CAD build for the part. Positions are in the model's coordinates, mm. A direction names the side the tool comes from. Give positions to 0.01 mm unless a question says otherwise; leave off trailing zeros. Order: outer loops, then holes, each group sorted by start corner. A loop starts at its lowest first (then second) coordinate and runs counter-clockwise, first axis right, second up. Notation, with made-up numbers: (16, 0) -> (73, 0) arc R16 cw to (73, 19) -> close; hole circle Ø4 at (45, 81). An arc over 180 degrees is marked (long way). Answer as CSV lines item,"result".
Autodesk Inventor part; units mm, degrees
ref_plane "YZ Plane" through (0, 0, 0) normal (1, 0, 0) x (0, 1, 0)
ref_plane "XZ Plane" through (0, 0, 0) normal (0, 1, 0) x (-1, 0, 0)
ref_plane "XY Plane" through (0, 0, 0) normal (0, 0, 1) x (1, 0, 0)
sketch "スケッチ1" plane through (0, 0, 0) normal (0, 0, 1) x (1, 0, 0)
  line L0 (0, 0) -> (3, 0)
  line L1 (3, 0) -> (3, -15)
  line L2 (3, -15) -> (0, -15)
  line L3 (0, -15) -> (0, 0)
  line L4 (-15, 0) -> (-12, 0)
  line L5 (-12, 0) -> (-12, -15)
  line L6 (-12, -15) -> (-15, -15)
  line L7 (-15, -15) -> (-15, 0)
  line L8 (-26.0926, 3) -> (-139.0635, -55.2952)
  line L9 (7, 3) -> (7, -18)
  line L10 (-7.8217, -18) -> (-133.786, -83)
  circle A0 centre (-135, -78) radius 2
  circle A1 centre (-150, -78) radius 2
  line L11 (-150, -78) -> (-135, -78) construction
  arc A2 (-154.0422, -75.0571) -> (-150, -83) centre (-150, -78) ccw
  line L12 (-140.638, -56.6456) -> (-154.0422, -75.0571)
  circle A3 centre (-15, -1.05) radius 1.05
  circle A4 centre (-15, -13.95) radius 1.05
  circle A5 centre (-12, -13.95) radius 1.05
  circle A6 centre (-12, -1.05) radius 1.05
  circle A7 centre (0, -1.05) radius 1.05
  circle A8 centre (3, -1.05) radius 1.05
  circle A9 centre (0, -13.95) radius 1.05
  circle A10 centre (3, -13.95) radius 1.05
  arc A11 (-139.0635, -55.2952) -> (-140.638, -56.6456) centre (-137, -59.2941) ccw
  circle A12 centre (-100.7273, -60.8773) radius 4.5 construction
  circle A13 centre (-81, -30.3971) radius 4.5 construction
  circle A14 centre (-44.7273, -31.9802) radius 4.5 construction
  circle A15 centre (-25, -1.5) radius 4.5 construction
  circle A16 centre (-137, -59.2941) radius 1.5
  circle A17 centre (-100.7273, -60.8773) radius 1.5
  circle A18 centre (-81, -30.3971) radius 1.5
  circle A19 centre (-44.7273, -31.9802) radius 1.5
  circle A20 centre (-25, -1.5) radius 1.5
  circle A21 centre (-4.5, -7.5) radius 1.5
  circle A22 centre (-19.5, -7.5) radius 1.5
  line L13 (-26.0926, 3) -> (7, 3)
  line L14 (-7.8217, -18) -> (7, -18)
  line L15 (-150, -83) -> (-133.786, -83)
  circle A23 centre (-135, -78) radius 5
  line L16 (-25, -1.5) -> (-44.7273, -31.9802) construction
  line L17 (-44.7273, -31.9802) -> (-81, -30.3971) construction
  line L18 (-81, -30.3971) -> (-100.7273, -60.8773) construction
  line L19 (-100.7273, -60.8773) -> (-137, -59.2941) construction
  point P0 (0, -12.9)
  point P1 (0, -2.1)
  point P2 (3, -2.1)
  point P3 (3, -12.9)
  point P4 (-12, -2.1)
  point P5 (-12, -12.9)
  point P6 (-15, -12.9)
  point P7 (-15, -2.1)
  dimension "d0" = 3
  dimension "d1" = 15
  dimension "d2" = 3
  dimension "d3" = 15
  dimension "d4" = 12
  dimension "d5" = 4
  dimension "d6" = 4
  dimension "d7" = 15
  dimension "d8" = 4
  dimension "d12" = 3
  dimension "d13" = 2.1
  dimension "d14" = 2.1
  dimension "d15" = 2.1
  dimension "d16" = 2.1
  dimension "d17" = 2.1
  dimension "d18" = 2.1
  dimension "d19" = 2.1
  dimension "d20" = 2.1
  dimension "d23" = 9
  dimension "d24" = 9
  dimension "d25" = 9
  dimension "d26" = 9
  dimension "d27" = 9
  dimension "d28" = 3
  dimension "d29" = 3
  dimension "d30" = 3
  dimension "d31" = 3
  dimension "d32" = 3
  dimension "d33" = 10
  dimension "d34" = 3
  dimension "d35" = 3
  dimension "d36" = 4.5
  dimension "d37" = 4.5
  dimension "d38" = 7.5
  dimension "d39" = 7.5
  dimension "d60" = 120
  dimension "d61" = 3
  dimension "d62" = 3
  dimension "d63" = 3
  dimension "d64" = 60
extrude "押し出し1" add sketch "スケッチ1" along normal blind 3
sketch "スケッチ3" plane through (0, 0, 3) normal (0, 0, 1) x (1, 0, 0)
  line L0 (-150, -83) -> (-133.786, -83)
  line L1 (-133.786, -83) -> (-7.8217, -18)
  line L2 (-7.8217, -18) -> (7, -18)
  line L3 (7, -18) -> (7, 3)
  line L4 (7, 3) -> (-26.0926, 3)
  line L5 (-26.0926, 3) -> (-139.0635, -55.2952)
  arc A0 (-139.0635, -55.2952) -> (-140.638, -56.6456) centre (-137, -59.2941) ccw
  line L6 (-140.638, -56.6456) -> (-154.0422, -75.0571)
  arc A1 (-154.0422, -75.0571) -> (-150, -83) centre (-150, -78) ccw
  circle A2 centre (-19.5, -7.5) radius 1.5
  circle A3 centre (-25, -1.5) radius 1.5
  circle A4 centre (-44.7273, -31.9802) radius 1.5
  circle A5 centre (-81, -30.3971) radius 1.5
  circle A6 centre (-100.7273, -60.8773) radius 1.5
  circle A7 centre (-137, -59.2941) radius 1.5
  arc A8 (3, -2.1) -> (3, 0) centre (3, -1.05) ccw
  line L7 (3, -2.1) -> (3, -12.9)
  arc A9 (3, -15) -> (3, -12.9) centre (3, -13.95) ccw
  line L8 (3, -15) -> (0, -15)
  arc A10 (0, -12.9) -> (0, -15) centre (0, -13.95) ccw
  line L9 (0, -12.9) -> (0, -2.1)
  arc A11 (0, 0) -> (0, -2.1) centre (0, -1.05) ccw
  line L10 (0, 0) -> (3, 0)
  circle A12 centre (-135, -78) radius 2
  line L11 (-12, -2.1) -> (-12, -12.9)
  arc A13 (-12, -15) -> (-12, -12.9) centre (-12, -13.95) ccw
  line L12 (-12, -15) -> (-15, -15)
  arc A14 (-15, -12.9) -> (-15, -15) centre (-15, -13.95) ccw
  line L13 (-15, -12.9) -> (-15, -2.1)
  arc A15 (-15, 0) -> (-15, -2.1) centre (-15, -1.05) ccw
  line L14 (-15, 0) -> (-12, 0)
  arc A16 (-12, -2.1) -> (-12, 0) centre (-12, -1.05) ccw
  circle A17 centre (-4.5, -7.5) radius 1.5
  circle A18 centre (-150, -78) radius 2
  line L15 (-137.6878, -57.9612) -> (-25.3642, 0)
  line L16 (-25.3642, 0) -> (4, 0)
  line L17 (4, 0) -> (4, -15)
  line L18 (4, -15) -> (-8.5501, -15)
  line L19 (-8.5501, -15) -> (-134.5144, -80)
  line L20 (-134.5144, -80) -> (-150, -80)
  arc A19 (-151.6169, -76.8229) -> (-150, -80) centre (-150, -78) ccw
  line L21 (-151.6169, -76.8229) -> (-138.2127, -58.4113)
  arc A20 (-137.6878, -57.9612) -> (-138.2127, -58.4113) centre (-137, -59.2941) ccw
  circle A21 centre (-81, -30.3971) radius 4.5
  circle A22 centre (-100.7273, -60.8773) radius 4.5
  circle A23 centre (-137, -59.2941) radius 4.5
  circle A24 centre (-44.7273, -31.9802) radius 4.5
  circle A25 centre (-19.5, -7.5) radius 4.5
  line L22 (-9, -11.2292) -> (-9, -3.7708)
  arc A26 (-9, -3.7708) -> (-12, 3) centre (-12, -1.05) ccw
  line L23 (-12, 3) -> (-15, 3)
  arc A27 (-15, 3) -> (-18, -3.7708) centre (-15, -1.05) ccw
  line L24 (-18, -3.7708) -> (-18, -11.2292)
  arc A28 (-18, -11.2292) -> (-15, -18) centre (-15, -13.95) ccw
  line L25 (-15, -18) -> (-12, -18)
  arc A29 (-12, -18) -> (-9, -11.2292) centre (-12, -13.95) ccw
  circle A30 centre (-25, -1.5) radius 4.5
  line L26 (-3, -3.7708) -> (-3, -11.2292)
  arc A31 (-3, -11.2292) -> (0, -18) centre (0, -13.95) ccw
  line L27 (0, -18) -> (3, -18)
  arc A32 (3, -18) -> (6, -11.2292) centre (3, -13.95) ccw
  line L28 (6, -11.2292) -> (6, -3.7708)
  arc A33 (6, -3.7708) -> (3, 3) centre (3, -1.05) ccw
  line L29 (3, 3) -> (0, 3)
  arc A34 (0, 3) -> (-3, -3.7708) centre (0, -1.05) ccw
  circle A35 centre (-4.5, -7.5) radius 4.6
  circle A36 centre (-135, -78) radius 5
  circle A37 centre (-150, -78) radius 5
  line L30 (-135, -73) -> (-150, -73)
  circle A38 centre (-137, -59.2941) radius 1.5
  line L31 (-137, -59.2941) -> (-100.7273, -60.8773) construction
  line L32 (-137.0654, -60.7927) -> (-100.7927, -62.3759)
  line L33 (-100.6619, -59.3787) -> (-136.9346, -57.7956)
  arc A39 (-136.9346, -57.7956) -> (-137.0654, -60.7927) centre (-137, -59.2941) ccw
  arc A40 (-100.7927, -62.3759) -> (-100.6619, -59.3787) centre (-100.7273, -60.8773) ccw
  line L34 (-81, -30.3971) -> (-100.7273, -60.8773) construction
  line L35 (-82.2593, -29.5821) -> (-101.9866, -60.0623)
  line L36 (-99.4681, -61.6923) -> (-79.7407, -31.2121)
  arc A41 (-79.7407, -31.2121) -> (-82.2593, -29.5821) centre (-81, -30.3971) ccw
  arc A42 (-101.9866, -60.0623) -> (-99.4681, -61.6923) centre (-100.7273, -60.8773) ccw
  line L37 (-81, -30.3971) -> (-44.7273, -31.9802) construction
  line L38 (-81.0654, -31.8956) -> (-44.7927, -33.4788)
  line L39 (-44.6619, -30.4816) -> (-80.9346, -28.8985)
  arc A43 (-80.9346, -28.8985) -> (-81.0654, -31.8956) centre (-81, -30.3971) ccw
  arc A44 (-44.7927, -33.4788) -> (-44.6619, -30.4816) centre (-44.7273, -31.9802) ccw
  line L40 (-25, -1.5) -> (-44.7273, -31.9802) construction
  line L41 (-26.2593, -0.685) -> (-45.9866, -31.1652)
  line L42 (-43.4681, -32.7952) -> (-23.7407, -2.315)
  arc A45 (-23.7407, -2.315) -> (-26.2593, -0.685) centre (-25, -1.5) ccw
  arc A46 (-45.9866, -31.1652) -> (-43.4681, -32.7952) centre (-44.7273, -31.9802) ccw
  point P0 (-118.8637, -60.0857)
  point P1 (-90.8637, -45.6372)
  point P2 (-62.8637, -31.1886)
  point P3 (-34.8637, -16.7401)
  point P4 (-3.5501, -12.0009)
  point P5 (-9, -8.4539)
  point P6 (-8.0885, -15)
  point P7 (-3.9115, -15)
  point P8 (-9, -6.5461)
  point P9 (-3.5501, -2.9991)
  point P10 (-3.9115, 0)
  point P11 (-8.0885, 0)
  point P12 (-26.046, -5.8768)
  point P13 (-41.1629, -29.2335)
  point P14 (-40.2692, -31.3677)
  point P15 (-14.3638, -18)
  point P16 (-18.4832, -11.8836)
  point P17 (-23.6655, -5.7976)
  point P18 (-43.6814, -27.6035)
  point P19 (-28.5645, -4.2467)
  point P20 (-29.4581, -2.1125)
  point P21 (-77.9176, -27.1186)
  point P22 (-76.696, -29.0835)
  point P23 (-48.9005, -30.2967)
  point P24 (-49.0314, -33.2938)
  point P25 (-76.8268, -32.0806)
  point P26 (-82.046, -34.7738)
  point P27 (-97.1629, -58.1306)
  point P28 (-96.2692, -60.2648)
  point P29 (-47.8098, -35.2587)
  point P30 (-99.6814, -56.5005)
  point P31 (-84.5645, -33.1438)
  point P32 (-85.4581, -31.0096)
  point P33 (-133.9176, -56.0156)
  point P34 (-132.696, -57.9806)
  point P35 (-104.9005, -59.1937)
  point P36 (-105.0314, -62.1909)
  point P37 (-132.8268, -60.9777)
  point P38 (-140.7098, -61.8412)
  point P39 (-148.8337, -73)
  point P40 (-130.0105, -77.6759)
  point P41 (-103.8098, -64.1558)
  dimension "d65" = 3
  dimension "d66" = 3
  dimension "d67" = 3
  dimension "d68" = 3
  dimension "d69" = 3
  dimension "d70" = 3
  dimension "d71" = 3
  dimension "d72" = 3
  dimension "d73" = 3
  dimension "d74" = 3.1
  dimension "d75" = 3
  dimension "d76" = 3
  dimension "d77" = 3
  dimension "d78" = 3
  dimension "d79" = 3
  dimension "d80" = 3
extrude "押し出し3" cut sketch "スケッチ3" against normal blind 3 contours L30 L21 A23 L32 A22 L19 A36 | L15 A21 L35 A22 L33 A23 | L19 A22 L36 A21 L38 A24 | L15 A30 L41 A24 L39 A21 | A24 L42 A30 A25 A28 L25 L19 | L18 A29 L22 A35 A31 | L16 A34 A35 L22 A26
properties part number "横回転カウンター根本" material "アルミニウム 7075"
1) Which spindle directions (+Z, -Z, +X, -X, +Y, -Y) get a long thin tool onto all of the face, cutting with end or side? Do faces 1 (the flat face through (0, -8, 1)), 2 (the flat face through (7, -7, 1)). Say none if no direction does.
Data:
face 1,"+Z, -Z"
face 2,"+Z, -Z, +X, +Y, -Y"
2) Band-saw the part on A-A, the plane y = -42. Write the cut outline in (x, z), then the cut area to 3 significant figures.
Data:
outline,"(-113.3, 0) -> (-106.76, 0) -> (-106.76, 3) -> (-113.3, 3) -> close; (-90.3, 0) -> (-86.72, 0) -> (-86.72, 3) -> (-90.3, 3) -> close; (-60.87, 0) -> (-54.33, 0) -> (-54.33, 3) -> (-60.87, 3) -> close"
area,"50.0 mm2"
3) Band-saw the part on B-B, the plane x = -90.5. Write the cut outline in (y, z).
Data:
outline,"(-60.66, 0) -> (-57.29, 0) -> (-57.29, 3) -> (-60.66, 3) -> close; (-47.84, 0) -> (-42.31, 0) -> (-42.31, 3) -> (-47.84, 3) -> close; (-33.61, 0) -> (-30.24, 0) -> (-30.24, 3) -> (-33.61, 3) -> close"
4) Band-saw the part on D-D, the plane z = 0.8. Give the number of separate pieces and of enclosed holes in the cut face, then the cut area to 3 significant figures.
Data:
separate pieces,"1"
enclosed holes,"18"
area,"2,010 mm2"
5) Pin check, flat tips, straight feed: P1, Ø5, axis at x = -25, y = -1.5, coming from the +Z side; P2, Ø1.5, axis at y = -6, z = 2, coming from the -X side; P3, Ø1.5, axis at y = -5.5, z = 1.5, coming from the -X side; P4, Ø1.5, axis at x = -7, z = 1.5, coming from the -Y side. Stop position of each tip, or through.
Data:
P1,"stops at z = 3"
P2,"stops at x = -44.99"
P3,"stops at x = -44.02"
P4,"stops at y = -18"
6) Pull direction Y, two halves, no side cores. Call faces 3 (the flat face through (-69.922, -50.045, 1.479)), 4 (the flat face through (-147.246, -65.722, 1.479)), 5 (the cylindrical face through (-136.474, -79.352, 1.479)): pulls with the +Y half, pulls with the -Y half, needs draft (parallel to the pull), parting line crosses it, or undercut.
Data:
face 3,"pulls with the -Y half"
face 4,"pulls with the +Y half"
face 5,"undercut"
7) Wall check: line 1 along X through (y, z) = (-53, 1.9); line 2 along X through (y, z) = (-14, 1.4); line 3 along X through (y, z) = (-0.5, 2.2). Give the ranges that are in metal, low to high. Write a range as [from, to].
Data:
line 1,"x = [-134.62, -128.07], [-97.42, -93.84], [-82.19, -75.65]"
line 2,"x = [-59.04, -52.49], [-34.88, -31.3], [-19.05, -16.05], [-10.95, -7.95], [-4.05, -1.05], [4.05, 7]"
line 3,"x = [-32.88, -26.12], [-23.88, -15.89], [-11.11, -7.99], [-4.01, -0.89], [3.89, 7]"
8) Band-saw the part on C-C, the plane y = -67. Write the cut outline in (x, z).
Data:
outline,"(-148.18, 0) -> (-144.47, 0) -> (-144.47, 3) -> (-148.18, 3) -> close; (-109.32, 0) -> (-102.78, 0) -> (-102.78, 3) -> (-109.32, 3) -> close"
